```python
from build123d import *

# Parameters (mm, degrees)
F0_R     = 18.5
F1_DEPTH = 26.924
F2_R     = 16.51
F3_DEPTH = 26.162
F5_DEPTH = 4.318
F6_R     = 3
F7_DEPTH = 18.161


with BuildPart() as f1:
    # F0 (on Top) → F1 (new body)
    with BuildSketch(Plane.XY):
        Circle(F0_R)
    extrude(amount=F1_DEPTH)

    # F2 (on face) → F3 (join)
    with BuildSketch(Plane(origin=(0, 0, 0), x_dir=(1, 0, 0), z_dir=(0, 0, -1))):
        Circle(F2_R)
    extrude(amount=F3_DEPTH)

    # F4 (on face) → F5 (join)
    with BuildSketch(Plane.XY.offset(26.924)):
        with BuildLine():
            ThreePointArc((5.969, -7.0954), (-4.22072, -2.87468), (0, -13.0644))
            ThreePointArc((0, -13.0644), (4.22072, -11.31612), (5.969, -7.0954))
        make_face()
    extrude(amount=F5_DEPTH)

    # F6 (on face) → F7 (join)
    with BuildSketch(Plane.XY.offset(31.242)):
        with Locations((0, -7.0954)):
            Circle(F6_R)
    extrude(amount=F7_DEPTH)


solid = f1.part
```
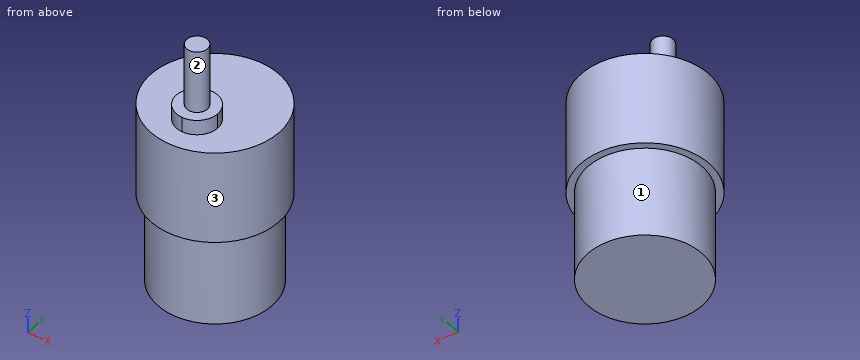
CAD build for the part. Positions are in the model's coordinates, mm. Face numbers are marked on the shaded views. A direction names the side the tool comes from. Round coordinates to 2 decimals unless told otherwise and drop trailing zeros. Loops run counter-clockwise (first coordinate to the right, second up) from the corner with the lowest first, then second, coordinate; pieces in that order, holes last. Notation, with made-up numbers: M -39.75,-29 L 11.25,-29 A21 cw 11.25,-7 Z; hole C -2.75,8.5 d11. An arc over 180 degrees is marked long. Use a Markdown table: item, result. Add a question column.
(1) Drill centre lines: line 1 (Z direction, x = 10, y = 13.5); line 2 (Z direction, x = -5.5, y = -2); line 3 (X direction, y = 5, z = 23). Where is each one in solid material? Low to high.
(2) Cut at D-D (x = -4). Give the cut face in (y, z), and give its area (3 significant figures).
(3) Cut at C-C (z = 28). Give the cut face in (x, y).
(4) Flat gauge pins, fed straight in: pin 1 (2 mm diameter, centred on x = 6, y = -9.5, fed in from +Z); pin 2 (1.5 mm diameter, centred on x = 2, z = 40.5, fed in from +Y); pin 3 (1.5 mm diameter, centred on x = 0.5, z = -9.5, fed in from +Y). Where does each tip first touch, or does it go through?
(5) Cut at A-A (y = 0). Give the cut face in (x, z).
(6) Cut at B-B (x = 13). Give the cut face in (y, z), and give its area (3 significant figures).
(7) Which spindle directions (+Z, -Z, +X, -X, +Y, -Y) get a long thin tool onto all of the face, cutting with end or side? Do the marked faces 1, 2 and 3. Say none if no direction does.
Geometry says:
| question | item | result |
|---|---|---|
| 1 | line 1 | z = 0 to 26.92 |
| 1 | line 2 | z = -26.16 to 26.92 |
| 1 | line 3 | x = -17.81 to 17.81 |
| 2 | outline | M -18.06,0 L -16.02,0 L -16.02,-26.16 L 16.02,-26.16 L 16.02,0 L 18.06,0 L 18.06,26.92 L -2.66,26.92 L -2.66,31.24 L -11.53,31.24 L -11.53,26.92 L -18.06,26.92 Z |
| 2 | area | 1,850 mm² |
| 3 | outline | M 0,-13.06 A5.97 ccw 5.97,-7.1 A5.97 ccw long Z |
| 4 | pin 1 | stops at z = 31.24 |
| 4 | pin 2 | stops at y = -4.37 |
| 4 | pin 3 | stops at y = 16.51 |
| 5 | outline | M -18.5,0 L -16.51,0 L -16.51,-26.16 L 16.51,-26.16 L 16.51,0 L 18.5,0 L 18.5,26.92 L -18.5,26.92 Z |
| 6 | outline | M -13.16,0 L -10.18,0 L -10.18,-26.16 L 10.18,-26.16 L 10.18,0 L 13.16,0 L 13.16,26.92 L -13.16,26.92 Z |
| 6 | area | 1,240 mm² |
| 7 | face 1 | -Z |
| 7 | face 2 | +Z |
| 7 | face 3 | +Z, -Z |
